Source: CAD feature listing. Evaluate the final solid. Frame: model axes, mm. Give positions to 0.01 mm unless a question says otherwise; leave off trailing zeros. Order: outer loops, then holes, each group sorted by start corner. A loop starts at its lowest first (then second) coordinate and runs counter-clockwise, first axis right, second up.
from build123d import *

# Parameters (mm, degrees)
SKETCH_1_W          = 20
SKETCH_1_H          = 14
EXTRUDE_1_DEPTH     = 60
CUT_EXTRUDE_1_REACH = 65.632
SKETCH_2_R          = 5
CUT_EXTRUDE_2_REACH = 64.418
SKETCH_3_R          = 2.05


with BuildPart() as part:
    # 草图1 → 凸台-拉伸1 (new body)
    with BuildSketch(Plane(origin=(0, 0, 0), x_dir=(1, 0, 0), z_dir=(0, 1, 0))):
        Rectangle(SKETCH_1_W, SKETCH_1_H)
    extrude(amount=EXTRUDE_1_DEPTH)

    # 草图2 → 切除-拉伸1 (cut, up to next)
    with BuildSketch(Plane.ZY.offset(10), mode=Mode.PRIVATE) as cut_extrude_1_sk1:
        with Locations((0, 30)):
            Circle(SKETCH_2_R)
    cut_extrude_1_tool1 = extrude(cut_extrude_1_sk1.sketch, amount=-CUT_EXTRUDE_1_REACH, mode=Mode.PRIVATE) & part.part
    add(cut_extrude_1_tool1.solids().sort_by_distance((-10, 30, 0))[0], mode=Mode.SUBTRACT)

    # 草图3 → 切除-拉伸2 (cut, up to next)
    with BuildSketch(Plane(origin=(0, 0, -7), x_dir=(-1, 0, 0), z_dir=(0, 0, -1)), mode=Mode.PRIVATE) as cut_extrude_2_sk1:
        with Locations((0, 45)):
            Circle(SKETCH_3_R)
    cut_extrude_2_tool1 = extrude(cut_extrude_2_sk1.sketch, amount=-CUT_EXTRUDE_2_REACH, mode=Mode.PRIVATE) & part.part
    # 草图3 → 切除-拉伸2 (cut, up to next)
    with BuildSketch(Plane(origin=(0, 0, -7), x_dir=(-1, 0, 0), z_dir=(0, 0, -1)), mode=Mode.PRIVATE) as cut_extrude_2_sk2:
        with Locations((0, 15)):
            Circle(SKETCH_3_R)
    cut_extrude_2_tool2 = extrude(cut_extrude_2_sk2.sketch, amount=-CUT_EXTRUDE_2_REACH, mode=Mode.PRIVATE) & part.part
    add(cut_extrude_2_tool1.solids().sort_by_distance((0, 45, -7))[0], mode=Mode.SUBTRACT)
    add(cut_extrude_2_tool2.solids().sort_by_distance((0, 15, -7))[0], mode=Mode.SUBTRACT)


solid = part.part
1) Section query A-A on z = 0. Output: boundary loops of the cut face in (x, y).
Checks:
outline: (-10, 0) - (10, 0) - (10, 25) - (-10, 25) - close; (-10, 35) - (10, 35) - (10, 60) - (-10, 60) - close; hole circle Ø4.1 at (0, 15); hole circle Ø4.1 at (0, 45)
2) Section query D-D on x = 3.5. Output: boundary loops of the cut face in (y, z).
Checks:
outline: (0, -7) - (60, -7) - (60, 7) - (0, 7) - close; hole circle Ø10 at (30, 0)
3) Pull-direction query (Y, two-part tool) for faces 1 (the face through (0, 60, 0)), 2 (the face through (0, 30, -7)), 3 (the face through (-0.14, 25.12, -1.08)); classes: +Y half, -Y half, draft (parallel to the pull), parting line (faces both ways), or undercut.
Checks:
face 1: +Y half
face 2: draft
face 3: undercut
4) Ray query, L1, parallel to Y at x = -1.75, z = -3; L2, parallel to Y at x = 0, z = -2.25; L3, parallel to Y at x = -5, z = -0.25. Return the intervals inside material, ascending.
Checks:
L1: y = 0 to 13.93, 16.07 to 26, 34 to 43.93, 46.07 to 60
L2: y = 0 to 12.95, 17.05 to 25.53, 34.47 to 42.95, 47.05 to 60
L3: y = 0 to 25.01, 34.99 to 60
5) First-contact query: pin 1 Ø6 at (y, z) = (30, 0) entering from -X. Flat tip, straight axial feed; report the tip coordinate or a pass-through.
Checks:
pin 1: passes through
6) Section query B-B on x = 0. Output: boundary loops of the cut face in (y, z), and give its area (3 significant figures).
Checks:
outline: (0, -7) - (12.95, -7) - (12.95, 7) - (0, 7) - close; (17.05, -7) - (42.95, -7) - (42.95, 7) - (17.05, 7) - close; (47.05, -7) - (60, -7) - (60, 7) - (47.05, 7) - close; hole circle Ø10 at (30, 0)
area: 647 mm2
7) Section query C-C on y = 15. Output: boundary loops of the cut face in (x, z).
Checks:
outline: (-10, -7) - (-2.05, -7) - (-2.05, 7) - (-10, 7) - close; (2.05, -7) - (10, -7) - (10, 7) - (2.05, 7) - close
